Could you check a few things on this model? Use its own coordinates, in mm. Coordinates: 2 decimals unless noted, no trailing zeros. Loops run counter-clockwise (first coordinate to the right, second up) from the corner with the lowest first, then second, coordinate; pieces in that order, holes last.
1) If I drill on line 1 along X through (y, z) = (492, 9); line 2 along Y through (x, z) = (-289.5, 8.75); line 3 along Y through (x, z) = (-1715, 1.25), over which ranges is the centre line in solid material (lowest first)?
2) Imagine slicing it at A-A on x = -267. Please give me the cut outline in (y, z).
3) Imagine slicing it at D-D on y = 131.5. Please give me the cut outline in (x, z).
4) Will these pins go through, and if not, where does the flat tip stop? P1, Ø12.5, axis at x = -1860, z = 18.5, coming from the -Y side; P2, Ø12.5, axis at x = -2124, z = 7.5, coming from the +Y side; P3, Ø7.5, axis at x = -2126, z = 16, coming from the -Y side.
5) Imagine slicing it at C-C on z = 14. Give the number of separate pieces and of enclosed holes in the cut face, plus the area to 3 significant figures.
6) Imagine slicing it at B-B on y = 685. Please give me the cut outline in (x, z).
```python
from build123d import *

# Parameters (mm, degrees)
SKETCH_W   = 657.016146
SKETCH_H   = 428
SKETCH_W_2 = 763
SKETCH_H_2 = 1068
PAD_DEPTH  = 25


with BuildPart() as part:
    # Sketch → Pad (new body)
    with BuildSketch(Plane.XY):
        Polygon((0, 0), (-813, 0), (-1395.667241, 39.432052), (-2335, 363), (-2360, 363), (-2360, 755), (-2335, 755), (-1395.667241, 1078.567948), (-813, 1118), (0, 1118), align=None)
        Polygon((-2335, 728.558359), (-2335, 389.441641), (-2205.983854, 345), (-2095, 345), (-2095, 773), (-2205.983854, 773), align=None, mode=Mode.SUBTRACT)
        with Locations((-1741.491927, 559)):
            Rectangle(SKETCH_W, SKETCH_H, mode=Mode.SUBTRACT)
        Polygon((-2133.407695, 798), (-1412.983854, 1046.161327), (-1412.983854, 798), align=None, mode=Mode.SUBTRACT)
        Polygon((-2133.407695, 320), (-1412.983854, 320), (-1412.983854, 71.838673), align=None, mode=Mode.SUBTRACT)
        Polygon((-1387.983854, 1054.030739), (-1387.983854, 63.969261), (-813, 25.057184), (-813, 1092.942816), align=None, mode=Mode.SUBTRACT)
        with Locations((-406.5, 559)):
            Rectangle(SKETCH_W_2, SKETCH_H_2, mode=Mode.SUBTRACT)
    extrude(amount=PAD_DEPTH)


solid = part.part
```
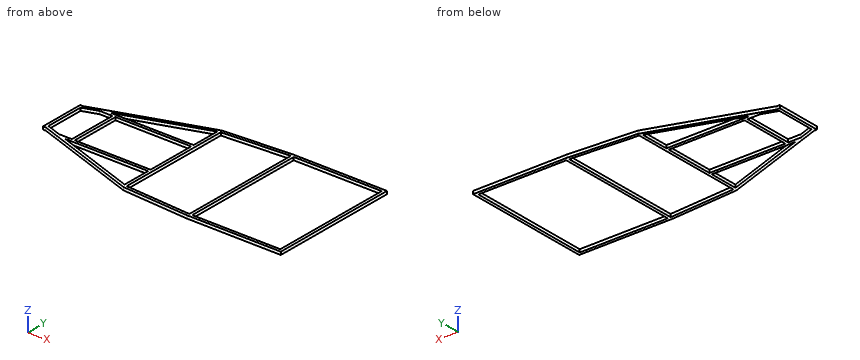
Filled in:
1. line 1: x = -2360 to -2335, -2095 to -2070, -1412.98 to -1387.98, -813 to -788, -25 to 0
1. line 2: y = 0 to 25, 1093 to 1118
1. line 3: y = 149.43 to 175.87, 320 to 345, 773 to 798, 942.13 to 968.57
2. outline: (0, 0) - (25, 0) - (25, 25) - (0, 25) - close; (1093, 0) - (1118, 0) - (1118, 25) - (1093, 25) - close
3. outline: (-1662.94, 0) - (-1586.18, 0) - (-1586.18, 25) - (-1662.94, 25) - close; (-1412.98, 0) - (-1387.98, 0) - (-1387.98, 25) - (-1412.98, 25) - close; (-813, 0) - (-788, 0) - (-788, 25) - (-813, 25) - close; (-25, 0) - (0, 0) - (0, 25) - (-25, 25) - close
4. P1: stops at y = 197.23
4. P2: stops at y = 829.84
4. P3: stops at y = 289.71
5. separate pieces: 1
5. enclosed holes: 6
5. area: 256,000 mm2
6. outline: (-2360, 0) - (-2335, 0) - (-2335, 25) - (-2360, 25) - close; (-2095, 0) - (-2070, 0) - (-2070, 25) - (-2095, 25) - close; (-1412.98, 0) - (-1387.98, 0) - (-1387.98, 25) - (-1412.98, 25) - close; (-813, 0) - (-788, 0) - (-788, 25) - (-813, 25) - close; (-25, 0) - (0, 0) - (0, 25) - (-25, 25) - close
